Autodesk Inventor part; units mm, degrees
ref_plane "YZ Plane" through (0, 0, 0) normal (1, 0, 0) x (0, 1, 0)
ref_plane "XZ Plane" through (0, 0, 0) normal (0, 1, 0) x (-1, 0, 0)
ref_plane "XY Plane" through (0, 0, 0) normal (0, 0, 1) x (1, 0, 0)
sketch "Sketch1" plane through (0, 0, 0) normal (0, 0, 1) x (1, 0, 0)
  circle A0 centre (0, 0) radius 2.5
  line L0 (0, 0) -> (-15.5714, 12.5511)
  line L1 (0, 0) -> (20, 0) construction
  line L2 (-15.5714, 12.5511) -> (-18.3421, 9.1137)
  line L3 (0, 0) -> (-10.3273, 2.6535)
  line L4 (0, 0) -> (22.7557, 0) construction
  line L5 (0, 0) -> (-10.6628, 0)
  line L6 (-4.786, 9.5283) -> (-22.3661, 23.6985)
  line L7 (-22.3661, 23.6985) -> (-20.7973, 25.6449)
  circle A1 centre (-20.7973, 25.6449) radius 2.5
  line L8 (-18.3421, 9.1137) -> (-10.3273, 2.6535)
  line L9 (-23.2502, 25.1624) -> (-25.4393, 36.2891)
  line L10 (-23.2502, 25.1624) -> (-11.9102, 25.1624) construction
  line L11 (-25.4393, 36.2891) -> (-22.9863, 36.7717)
  circle A2 centre (-22.9863, 36.7717) radius 2.5
  line L12 (-25.0727, 38.149) -> (-21.9049, 42.9477)
  line L13 (-25.0727, 38.149) -> (-19.3227, 38.149) construction
  line L14 (-21.9049, 42.9477) -> (-23.9913, 44.325)
  circle A3 centre (-23.9913, 44.325) radius 2.5
  line L15 (0, 0) -> (60, 0) construction
  line L16 (-25.2189, 49.3225) -> (-22.1589, 46.0257)
  line L17 (-23.9913, 39.7871) -> (-31.8111, 44.9492)
  line L18 (-31.8111, 44.9492) -> (-29.1376, 48.9991)
  line L19 (-31.8111, 44.9492) -> (-34.1674, 41.3798)
  line L20 (-24.1412, 29.6912) -> (-32.2851, 28.089)
  line L21 (-32.2851, 28.089) -> (-34.534, 39.5199)
  line L22 (-32.2851, 28.089) -> (-30.6518, 19.787)
  line L23 (-18.3421, 9.1137) -> (-29.7677, 18.3232)
  line L24 (-18.3421, 20.455) -> (-23.8834, 13.5802)
  arc A4 (-12.5406, 2.5003) -> (-12.6967, 1.5208) centre (-12.5054, 1.9925) ccw
  line L25 (-10.3273, 2.6535) -> (-12.5406, 2.5003)
  line L26 (-10.6406, 0.6873) -> (-12.6967, 1.5208)
  line L27 (-10.6455, -0.6061) -> (-12.7079, -1.4239)
  line L28 (-10.3473, -2.5746) -> (-12.5593, -2.4045)
  arc A5 (-12.7079, -1.4239) -> (-12.5593, -2.4045) centre (-12.5203, -1.897) ccw
  line L29 (-9.9594, -3.8085) -> (-11.6763, -5.2137)
  line L30 (-9.0777, -5.5937) -> (-11.2371, -6.103)
  arc A6 (-11.6763, -5.2137) -> (-11.2371, -6.103) centre (-11.3539, -5.6076) ccw
  line L31 (-8.3337, -6.6517) -> (-9.5431, -8.5116)
  line L32 (-6.9518, -8.085) -> (-8.8547, -9.2257)
  arc A7 (-9.5431, -8.5116) -> (-8.8547, -9.2257) centre (-9.1164, -8.7891) ccw
  line L33 (-5.9217, -8.8672) -> (-6.5096, -11.0065)
  line L34 (-4.17, -9.8136) -> (-5.6369, -11.478)
  arc A8 (-6.5096, -11.0065) -> (-5.6369, -11.478) centre (-6.0188, -11.1414) ccw
  line L35 (-2.951, -10.2463) -> (-2.8619, -12.4631)
  line L36 (-0.9947, -10.6163) -> (-1.8873, -12.6474)
  arc A9 (-2.8619, -12.4631) -> (-1.8873, -12.6474) centre (-2.3533, -12.4426) ccw
  line L37 (0.298, -10.6586) -> (1.0558, -12.7438)
  line L38 (2.2743, -10.4174) -> (2.0403, -12.6236)
  arc A10 (1.0558, -12.7438) -> (2.0403, -12.6236) centre (1.5342, -12.5699) ccw
  line L39 (3.5189, -10.0654) -> (4.8738, -11.8222)
  line L40 (5.3288, -9.2357) -> (5.7755, -11.4089)
  arc A11 (4.8738, -11.8222) -> (5.7755, -11.4089) centre (5.2769, -11.5113) ccw
  line L41 (6.4079, -8.5225) -> (8.2321, -9.7852)
  line L42 (7.8806, -7.1827) -> (8.9658, -9.1178)
  arc A12 (8.2321, -9.7852) -> (8.9658, -9.1178) centre (8.5218, -9.3667) ccw
  line L43 (8.6923, -6.1756) -> (10.8137, -6.8251)
  line L44 (9.6889, -4.452) -> (11.3102, -5.9665)
  arc A13 (10.8137, -6.8251) -> (11.3102, -5.9665) centre (10.9627, -6.3384) ccw
  line L45 (10.1566, -3.2461) -> (12.3751, -3.2211)
  line L46 (10.5831, -1.3013) -> (12.5875, -2.2522)
  arc A14 (12.3751, -3.2211) -> (12.5875, -2.2522) centre (12.3693, -2.7121) ccw
  line L47 (10.6628, -0.0103) -> (12.769, 0.6868)
  line L48 (10.4788, 1.9721) -> (12.6773, 1.6744)
  arc A15 (12.769, 0.6868) -> (12.6773, 1.6744) centre (12.609, 1.17) ccw
  line L49 (10.1629, 3.2264) -> (11.9582, 4.5299)
  line L50 (9.3859, 5.0595) -> (11.5711, 5.4432)
  arc A16 (11.9582, 4.5299) -> (11.5711, 5.4432) centre (11.6591, 4.9418) ccw
  line L51 (8.7043, 6.1588) -> (10.0192, 7.9457)
  line L52 (7.4075, 7.6696) -> (9.3732, 8.6983)
  arc A17 (10.0192, 7.9457) -> (9.3732, 8.6983) centre (9.6092, 8.2474) ccw
  line L53 (6.4244, 8.5101) -> (7.135, 10.6118)
  line L54 (4.7303, 9.5561) -> (6.291, 11.1329)
  arc A18 (7.135, 10.6118) -> (6.291, 11.1329) centre (6.6528, 10.7748) ccw
  line L55 (3.5385, 10.0585) -> (3.5776, 12.2768)
  line L56 (1.6068, 10.541) -> (2.6153, 12.5171)
  arc A19 (3.5776, 12.2768) -> (2.6153, 12.5171) centre (3.0687, 12.2857) ccw
  line L57 (0.3187, 10.658) -> (-0.3173, 12.7835)
  line L58 (-1.6683, 10.5314) -> (-1.3071, 12.7204)
  arc A20 (-0.3173, 12.7835) -> (-1.3071, 12.7204) centre (-0.8049, 12.6376) ccw
  line L59 (-2.9312, 10.252) -> (-4.1823, 12.0842)
  line L60 (-4.786, 9.5283) -> (-5.1063, 11.7237)
  arc A21 (-4.1823, 12.0842) -> (-5.1063, 11.7237) centre (-4.6026, 11.7971) ccw
  arc A22 (-1.6683, 10.5314) -> (-2.9312, 10.252) centre (0, 0) ccw
  arc A23 (1.6068, 10.541) -> (0.3187, 10.658) centre (0, 0) ccw
  arc A24 (4.7303, 9.5561) -> (3.5385, 10.0585) centre (0, 0) ccw
  arc A25 (7.4075, 7.6696) -> (6.4244, 8.5101) centre (0, 0) ccw
  arc A26 (9.3859, 5.0595) -> (8.7043, 6.1588) centre (0, 0) ccw
  arc A27 (10.4788, 1.9721) -> (10.1629, 3.2264) centre (0, 0) ccw
  arc A28 (10.5831, -1.3013) -> (10.6628, 0) centre (0, 0) ccw
  arc A29 (9.6889, -4.452) -> (10.1566, -3.2461) centre (0, 0) ccw
  arc A30 (7.8806, -7.1827) -> (8.6923, -6.1756) centre (0, 0) ccw
  arc A31 (5.3288, -9.2357) -> (6.4079, -8.5225) centre (0, 0) ccw
  arc A32 (2.2743, -10.4174) -> (3.5189, -10.0654) centre (0, 0) ccw
  arc A33 (-0.9947, -10.6163) -> (0.298, -10.6586) centre (0, 0) ccw
  arc A34 (-4.17, -9.8136) -> (-2.951, -10.2463) centre (0, 0) ccw
  arc A35 (-6.9518, -8.085) -> (-5.9217, -8.8672) centre (0, 0) ccw
  arc A36 (-9.0777, -5.5937) -> (-8.3337, -6.6517) centre (0, 0) ccw
  arc A37 (-10.3473, -2.5746) -> (-9.9594, -3.8085) centre (0, 0) ccw
  arc A38 (-10.2331, 2.9964) -> (-10.3273, 2.6535) centre (0, 0) ccw
  arc A39 (-10.6406, 0.6873) -> (-10.6455, -0.6061) centre (0, 0) ccw
  line L61 (-4.9971, 9.2664) -> (-4.786, 9.5283)
  arc A40 (-25.2189, 49.3225) -> (-29.1376, 48.9991) centre (-27.0512, 47.6218) ccw
  arc A41 (-34.1674, 41.3798) -> (-34.534, 39.5199) centre (-32.081, 40.0025) ccw
  arc A42 (-30.6518, 19.787) -> (-29.7677, 18.3232) centre (-28.1988, 20.2696) ccw
  point P0 (-4.786, 9.5283)
  dimension "d0" = 5
  dimension "d1" = 20
  dimension "d2" = 141.13
  dimension "d3" = 4.415
  dimension "d4" = 165.59
  dimension "d5" = 22.58
  dimension "d6" = 2.5
  dimension "d10" = 11.34
  dimension "d12" = 101.13
  dimension "d13" = 2.5
  dimension "d15" = 5.75
  dimension "d17" = 56.57
  dimension "d18" = 2.5
  dimension "d22" = 9.37
  dimension "d23" = 8.3
  dimension "d24" = 8.83
  dimension "d25" = 1.991
  dimension "d27" = 1.018
  dimension "d30" = 300.366
  dimension "d32" = 2.5
extrude "Extrusion1" add sketch "Sketch1" along normal blind 4 contours A0 L0 L2 L23 L24 L6 L60 A21 L59 A22 L58 A20 L57 A23 L56 A19 L55 A24 L54 A18 L53 A25 L52 A17 L51 A26 L50 A16 L49 A27 L48 A15 L47 A28 L46 A14 L45 A29 L44 A13 L43 A30 L42 A12 L41 A31 L40 A11 L39 A32 L38 A10 L37 A33 L36 A9 L35 A34 L34 A8 L33 A35 L32 A7 L31 A36 L30 A6 L29 A37 L28 A5 L27 A39 L5 | A0 L3 L8 L2 L0 | L5 A39 L26 A4 L25 L3 A0 | L23 A42 L22 L20 L9 A1 L6 L24 | L21 A41 L19 L17 L12 A2 L9 L20 | L18 A40 L16 A3 L12 L17 | A3
properties part number "Servo pinza 1"
The model under review builds one solid part; all positions refer to its coordinate system, in mm. A direction names the side the tool comes from. Round coordinates to 2 decimals unless told otherwise and drop trailing zeros. Order: outer loops, then holes, each group sorted by start corner. A loop starts at its lowest first (then second) coordinate and runs counter-clockwise, first axis right, second up. Notation, with made-up numbers: (45.5, 77) -> (86.5, 77) arc R20 ccw to (86.5, 94) -> close; hole circle Ø10 at (38.25, 85). An arc over 180 degrees is marked (long way). Return JSON: item names as keys, results as strings.
1. Insertion check: P1, Ø2, axis at x = -9, z = 2.5, coming from the -Y side; P2, Ø2, axis at y = 18, z = 2, coming from the +X side. Each pin has a flat end and moves straight along its axis. Give the tip position at first contact, or say it passes through.
Answer block:
{"P1": "stops at y = -9.3", "P2": "stops at x = -14.06"}
2. The part is to be moulded in two halves that separate along Y. For faces 1 (the face through (-23.71, 47.697, 1.972)), 2 (the face through (-0.54, 2.44, 1.97)), 3 (the face through (-34.536, 40.473, 1.972)), 4 (the face through (-10.663, 0.032, 1.972)), say which applies: +Y half, -Y half, draft (parallel to the pull), parting line (faces both ways), or undercut.
Answer block:
{"face 1": "+Y half", "face 2": "undercut", "face 3": "parting line", "face 4": "undercut"}
3. For L1, parallel to X at y = 11, z = 1.25; L2, parallel to Y at x = -3, z = 0.55; L3, parallel to X at y = 44, z = 0.6, list the stretches that pass through material, from the lowest coordinate up. Write a range as [from, to].
Answer block:
{"L1": "x = [-20.68, -6.61], [-5, -3.44], [-1.59, 0.22], [1.84, 3.56], [6.16, 7.11]", "L2": "y = [-10.23, 10.35]", "L3": "x = [-32.44, -21.51]"}
4. For faces 5 (the face through (-11.44, -2.49, 1.97)), 6 (the face through (-7.89, -8.647, 1.972)), 7 (the face through (10.46, 5.25, 1.97)), 8 (the face through (5.5, 10.333, 1.972)), list the 3-axis set-ups (+Z, -Z, +X, -X, +Y, -Y) from which the entire face can be reached by the end or side of a thin tool; tool diameter is ignored.
Answer block:
{"face 5": "+Z, -Z, -X", "face 6": "+Z, -Z, -Y", "face 7": "+Z, -Z", "face 8": "+Z, -Z, +Y"}
5. Take a section at A-A (y = 27). Write out the cut boundary in (x, z), then the cut area to 3 significant figures.
Answer block:
{"outline": "(-32.07, 0) -> (-23.61, 0) -> (-23.61, 4) -> (-32.07, 4) -> close", "area": "33.8 mm²"}
6. Take a section at B-B (y = 17). Write out the cut boundary in (x, z).
Answer block:
{"outline": "(-28.13, 0) -> (-14.06, 0) -> (-14.06, 4) -> (-28.13, 4) -> close"}
